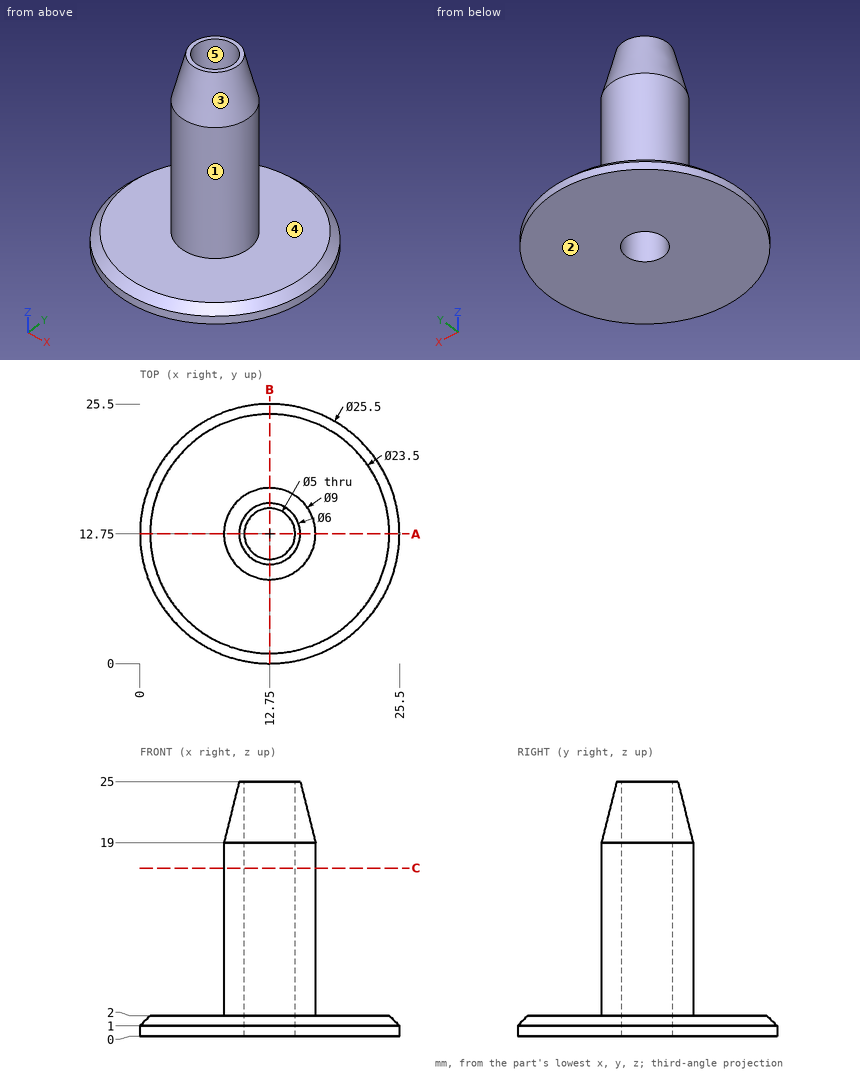
Could you check a few things on this drawing? It's one solid part, dimensions in mm from its lowest x, y, z. A direction names the side the tool comes from. Round coordinates to 2 decimals unless told otherwise and drop trailing zeros. Write each loop counter-clockwise with the first axis right and the second up, starting at its lowest first coordinate (ties: lowest second). Pieces come first, ordered by that corner, then holes. Notation, with made-up numbers: (59, 5.25) -> (79, 5.25) arc R6 cw to (79, 13.25) -> close; hole circle Ø3 at (79.25, -36.5). An arc over 180 degrees is marked (long way). Use a Markdown table: item, result.
1. For pin 1 Ø6 at (y, z) = (16.5, 18) entering from -X; pin 2 Ø10 at (x, y) = (15.5, 15.5) entering from -Z; pin 3 Ø6 at (x, z) = (16, 20.5) entering from +Y; pin 4 Ø4 at (x, z) = (9, 20) entering from +Y, each with a flat end and sliding along its axis, tell me the tip position at first contact or that it passes through.
Answer key:
| item | result |
|---|---|
| pin 1 | stops at x = 8.31 |
| pin 2 | stops at z = 0 |
| pin 3 | stops at y = 17.2 |
| pin 4 | stops at y = 16.77 |
2. If we section it at A-A (y = 12.75): List the corners of the cut face in (x, z) for me, then the cut area to 3 significant figures.
Answer key:
| item | result |
|---|---|
| outline | (0, 0) -> (10.25, 0) -> (10.25, 25) -> (9.75, 25) -> (8.25, 19) -> (8.25, 2) -> (1, 2) -> (0, 1) -> close; (15.25, 0) -> (25.5, 0) -> (25.5, 1) -> (24.5, 2) -> (17.25, 2) -> (17.25, 19) -> (15.75, 25) -> (15.25, 25) -> close |
| area | 123 mm^2 |
3. We'd pull the mould along Y, two halves only. Please class the marked faces 3, 4 and 5: +Y half, -Y half, draft (parallel to the pull), parting line (faces both ways), or undercut.
Answer key:
| item | result |
|---|---|
| face 3 | parting line |
| face 4 | draft |
| face 5 | undercut |
4. Which directions (+Z, -Z, +X, -X, +Y, -Y) give clear straight access to the entire face, cutting with the end or side of a thin tool? Please do the marked faces 1 and 2.
Answer key:
| item | result |
|---|---|
| face 1 | +Z |
| face 2 | -Z, +X, -X, +Y, -Y |
5. Please list where these lines run through material, in increasing order: probe 1 along Y at (x, z) = (12.75, 13.5); probe 2 along Z at (x, y) = (16, 2); probe 3 along Y at (x, z) = (12.75, 19.5) (3 decimals).
Answer key:
| item | result |
|---|---|
| probe 1 | y = 8.25 to 10.25, 15.25 to 17.25 |
| probe 2 | z = 0 to 2 |
| probe 3 | y = 8.375 to 10.25, 15.25 to 17.125 |
6. If we section it at C-C (z = 16.5): List the corners of the cut face in (x, y) for me.
Answer key:
| item | result |
|---|---|
| outline | circle Ø9 at (12.75, 12.75); hole circle Ø5 at (12.75, 12.75) |
